The model under review builds one solid part; all positions refer to its coordinate system, in mm. A direction names the side the tool comes from. Give positions to 0.01 mm unless a question says otherwise; leave off trailing zeros. Order: outer loops, then holes, each group sorted by start corner. A loop starts at its lowest first (then second) coordinate and runs counter-clockwise, first axis right, second up.
```python
from build123d import *

# Parameters (mm, degrees)
BOSS_EXTRUDE11_DEPTH = 10
BOSS_EXTRUDE12_DEPTH = 2
BOSS_EXTRUDE15_START = -8
BOSS_EXTRUDE15_DEPTH = 2
BOSS_EXTRUDE19_START = -10
SKETCH1_20_W         = 1.25
SKETCH1_20_H         = 3.5
BOSS_EXTRUDE19_DEPTH = 10
BOSS_EXTRUDE20_START = -20
SKETCH1_21_W         = 197.5
SKETCH1_21_H         = 3.5
BOSS_EXTRUDE20_DEPTH = 2
CUT_EXTRUDE1_REACH   = 249.148
SKETCH2_R            = 2.5
SKETCH2_3_R          = 6
SKETCH2_3_R_2        = 2.5
CUT_EXTRUDE2_DEPTH   = 4.75
CUT_EXTRUDE3_REACH   = 249.625
SKETCH3_R            = 2.5
SKETCH3_3_R          = 6
SKETCH3_3_R_2        = 2.5
CUT_EXTRUDE4_DEPTH   = 4.75


with BuildPart() as part:
    # Sketch1 → Boss-Extrude11 (new body)
    with BuildSketch(Plane.XY):
        with BuildLine():
            Line((201.25, 4.75), (201.25, 27.25))
            Line((201.25, 27.25), (1.25, 27.25))
            Line((1.25, 27.25), (1.25, 30.75))
            Line((1.25, 30.75), (226.5, 30.75))
            ThreePointArc((226.5, 30.75), (243, 14.25), (226.5, -2.25))
            Line((226.5, -2.25), (210, -2.25))
            Line((210, -2.25), (210, -3.5))
            Line((210, -3.5), (244.25, -3.5))
            Line((244.25, -3.5), (244.25, 32))
            Line((244.25, 32), (0, 32))
            Line((0, 32), (0, 26))
            Line((0, 26), (200, 26))
            Line((200, 26), (200, 6))
            Line((200, 6), (0, 6))
            Line((0, 6), (0, 0))
            Line((0, 0), (208.75, 0))
            Line((208.75, 0), (208.75, 1.25))
            Line((208.75, 1.25), (1.25, 1.25))
            Line((1.25, 1.25), (1.25, 4.75))
            Line((1.25, 4.75), (201.25, 4.75))
        make_face()
    extrude(amount=-BOSS_EXTRUDE11_DEPTH)

    # Sketch1<12> → Boss-Extrude12 (add)
    with BuildSketch(Plane.XY):
        with BuildLine():
            Line((201.25, 4.75), (1.25, 4.75))
            Line((1.25, 4.75), (1.25, 1.25))
            Line((1.25, 1.25), (208.75, 1.25))
            Line((208.75, 1.25), (208.75, 0))
            Line((208.75, 0), (210, 0))
            Line((210, 0), (210, -2.25))
            Line((210, -2.25), (226.5, -2.25))
            ThreePointArc((226.5, -2.25), (210, 14.25), (226.5, 30.75))
            Line((226.5, 30.75), (1.25, 30.75))
            Line((1.25, 30.75), (1.25, 27.25))
            Line((1.25, 27.25), (201.25, 27.25))
            Line((201.25, 27.25), (201.25, 4.75))
        make_face()
    extrude(amount=-BOSS_EXTRUDE12_DEPTH)

    # Sketch1<14> → Boss-Extrude15 (add)
    with BuildSketch(Plane.XY.offset(BOSS_EXTRUDE15_START)):
        with BuildLine():
            Line((201.25, 4.75), (198.75, 4.75))
            Line((198.75, 4.75), (198.75, 1.25))
            Line((198.75, 1.25), (208.75, 1.25))
            Line((208.75, 1.25), (208.75, 0))
            Line((208.75, 0), (210, 0))
            Line((210, 0), (210, -2.25))
            Line((210, -2.25), (226.5, -2.25))
            ThreePointArc((226.5, -2.25), (243, 14.25), (226.5, 30.75))
            Line((226.5, 30.75), (198.75, 30.75))
            Line((198.75, 30.75), (198.75, 27.25))
            Line((198.75, 27.25), (201.25, 27.25))
            Line((201.25, 27.25), (201.25, 4.75))
        make_face()
    extrude(amount=-BOSS_EXTRUDE15_DEPTH)

    # Sketch1<20> → Boss-Extrude19 (add)
    with BuildSketch(Plane.XY.offset(BOSS_EXTRUDE19_START)):
        Polygon((0, 26), (200, 26), (200, 27.25), (198.75, 27.25), (1.25, 27.25), (1.25, 30.75), (198.75, 30.75), (200, 30.75), (200, 32), (0, 32), align=None)
        with Locations((199.375, 29)):
            Rectangle(SKETCH1_20_W, SKETCH1_20_H)
        with Locations((199.375, 3)):
            Rectangle(SKETCH1_20_W, SKETCH1_20_H)
        Polygon((200, 4.75), (200, 6), (0, 6), (0, 0), (200, 0), (200, 1.25), (198.75, 1.25), (1.25, 1.25), (1.25, 4.75), (198.75, 4.75), align=None)
    extrude(amount=-BOSS_EXTRUDE19_DEPTH)

    # Sketch1<21> → Boss-Extrude20 (add)
    with BuildSketch(Plane.XY.offset(BOSS_EXTRUDE20_START)):
        with Locations((100, 3)):
            Rectangle(SKETCH1_21_W, SKETCH1_21_H)
        with Locations((100, 29)):
            Rectangle(SKETCH1_21_W, SKETCH1_21_H)
    extrude(amount=BOSS_EXTRUDE20_DEPTH)

    # Cut-Extrude1: up to this face of the body (flat: up to its plane)
    cut_extrude1_end = Plane(part.part.faces().sort_by_distance((100, 6, -10))[0])
    # Sketch2 → Cut-Extrude1 (cut, up to the picked face)
    with BuildSketch(Plane.XZ, mode=Mode.PRIVATE) as cut_extrude1_sk1:
        with Locations((32.5, -10)):
            Circle(SKETCH2_R)
    cut_extrude1_tool1 = split(extrude(cut_extrude1_sk1.sketch, amount=-CUT_EXTRUDE1_REACH, mode=Mode.PRIVATE), bisect_by=cut_extrude1_end, keep=Keep.BOTH, mode=Mode.PRIVATE)
    # Sketch2 → Cut-Extrude1 (cut, up to the picked face)
    with BuildSketch(Plane.XZ, mode=Mode.PRIVATE) as cut_extrude1_sk2:
        with Locations((155, -10)):
            Circle(SKETCH2_R)
    cut_extrude1_tool2 = split(extrude(cut_extrude1_sk2.sketch, amount=-CUT_EXTRUDE1_REACH, mode=Mode.PRIVATE), bisect_by=cut_extrude1_end, keep=Keep.BOTH, mode=Mode.PRIVATE)
    add(cut_extrude1_tool1.solids().sort_by(Axis((32.5, 0, -10), (0, 1, 0)))[0], mode=Mode.SUBTRACT)
    add(cut_extrude1_tool2.solids().sort_by(Axis((155, 0, -10), (0, 1, 0)))[0], mode=Mode.SUBTRACT)

    # Sketch2<3> → Cut-Extrude2 (cut)
    # profile 1 of 2: a face of its own
    with BuildSketch(Plane.XZ):
        with Locations(Location((155, -10, 0), (0, 0, 270))):
            Circle(SKETCH2_3_R)
        with Locations((155, -10)):
            Circle(SKETCH2_3_R_2, mode=Mode.SUBTRACT)
    # profile 2 of 2: a face of its own
    with BuildSketch(Plane.XZ):
        with Locations(Location((32.5, -10, 0), (0, 0, 270))):
            Circle(SKETCH2_3_R)
        with Locations((32.5, -10)):
            Circle(SKETCH2_3_R_2, mode=Mode.SUBTRACT)
    extrude(amount=-CUT_EXTRUDE2_DEPTH, mode=Mode.SUBTRACT)

    # Cut-Extrude3: up to this face of the body (flat: up to its plane)
    cut_extrude3_end = Plane(part.part.faces().sort_by_distance((100, 26, -10))[0])
    # Sketch3 → Cut-Extrude3 (cut, up to the picked face)
    with BuildSketch(Plane(origin=(0, 32, 0), x_dir=(1, 0, 0), z_dir=(0, 1, 0)), mode=Mode.PRIVATE) as cut_extrude3_sk1:
        with Locations(Location((157.5, 10, 0), (0, 0, 180))):
            Circle(SKETCH3_R)
    cut_extrude3_tool1 = split(extrude(cut_extrude3_sk1.sketch, amount=-CUT_EXTRUDE3_REACH, mode=Mode.PRIVATE), bisect_by=cut_extrude3_end, keep=Keep.BOTH, mode=Mode.PRIVATE)
    # Sketch3 → Cut-Extrude3 (cut, up to the picked face)
    with BuildSketch(Plane(origin=(0, 32, 0), x_dir=(1, 0, 0), z_dir=(0, 1, 0)), mode=Mode.PRIVATE) as cut_extrude3_sk2:
        with Locations(Location((55, 10, 0), (0, 0, 180))):
            Circle(SKETCH3_R)
    cut_extrude3_tool2 = split(extrude(cut_extrude3_sk2.sketch, amount=-CUT_EXTRUDE3_REACH, mode=Mode.PRIVATE), bisect_by=cut_extrude3_end, keep=Keep.BOTH, mode=Mode.PRIVATE)
    add(cut_extrude3_tool1.solids().sort_by(Axis((157.5, 32, -10), (0, -1, 0)))[0], mode=Mode.SUBTRACT)
    add(cut_extrude3_tool2.solids().sort_by(Axis((55, 32, -10), (0, -1, 0)))[0], mode=Mode.SUBTRACT)

    # Sketch3<3> → Cut-Extrude4 (cut)
    # profile 1 of 2: a face of its own
    with BuildSketch(Plane(origin=(0, 32, 0), x_dir=(1, 0, 0), z_dir=(0, 1, 0))):
        with Locations(Location((157.5, 10, 0), (0, 0, 180))):
            Circle(SKETCH3_3_R)
        with Locations(Location((157.5, 10, 0), (0, 0, 180))):
            Circle(SKETCH3_3_R_2, mode=Mode.SUBTRACT)
    # profile 2 of 2: a face of its own
    with BuildSketch(Plane(origin=(0, 32, 0), x_dir=(1, 0, 0), z_dir=(0, 1, 0))):
        with Locations(Location((55, 10, 0), (0, 0, 180))):
            Circle(SKETCH3_3_R)
        with Locations(Location((55, 10, 0), (0, 0, 180))):
            Circle(SKETCH3_3_R_2, mode=Mode.SUBTRACT)
    extrude(amount=-CUT_EXTRUDE4_DEPTH, mode=Mode.SUBTRACT)


solid = part.part
```
1. Take a section at A-A (x = 55). Write out the cut boundary in (y, z).
2. Take a section at C-C (y = 14.25). Write out the cut boundary in (x, z), and give its area (3 significant figures).
3. Take a section at B-B (x = 175). Write out the cut boundary in (y, z), and give its area (3 significant figures).
4. Draft analysis for pull direction Z (two halves, no side actions). For faces 1 (the flat face through (104, 0, -10)), 2 (the flat face through (222, 14, -10)), 3 (the cylindrical face through (155.19, 26.63, -10.96)), 4 (the flat face through (221, 14, -8)), state which applies: pulls with the +Z half, pulls with the -Z half, needs draft (parallel to the pull), parting line crosses it, or undercut.
5. For faces 5 (the cylindrical face through (31.96, 5.37, -12.44)), 6 (the cylindrical face through (61, 31, -10)), 7 (the flat face through (103, 27.25, -10)), list the 3-axis set-ups (+Z, -Z, +X, -X, +Y, -Y) from which the entire face can be reached by the end or side of a thin tool; tool diameter is ignored.
6. To check wall thickness, follow line 1 (Y direction, x = 84, z = -15.75); line 2 (Y direction, x = 149.5, z = -8.5); line 3 (Y direction, x = 29.5, z = -18.75). State the ranges of each line that lie inside material, in increasing order.
7. Insertion check: pin 1 (8 mm diameter, centred on x = 43.5, z = -10, fed in from -Y); pin 2 (1.5 mm diameter, centred on y = 5.5, z = -10.5, fed in from -X); pin 3 (1.8 mm diameter, centred on y = 28.5, z = -12, fed in from +X); pin 4 (11 mm diameter, centred on x = 155, z = -10, fed in from -Y). Each pin has a flat end and moves straight along its axis. Give the tip position at first contact, or say it passes through.
Answer:
1. outline: (0, -20) - (6, -20) - (6, 0) - (0, 0) - close; (26, -20) - (32, -20) - (32, -16) - (30.75, -16) - (30.75, -18) - (27.25, -18) - (27.25, -12.5) - (26, -12.5) - close; (26, -7.5) - (27.25, -7.5) - (27.25, -2) - (30.75, -2) - (30.75, -4) - (32, -4) - (32, 0) - (26, 0) - close; hole (1.25, -18) - (4.75, -18) - (4.75, -2) - (1.25, -2) - close
2. outline: (200, -10) - (244.25, -10) - (244.25, 0) - (243, 0) - (243, -8) - (201.25, -8) - (201.25, -2) - (210, -2) - (210, 0) - (200, 0) - close
2. area: 126 mm2
3. outline: (0, -20) - (6, -20) - (6, 0) - (0, 0) - close; (26, -20) - (32, -20) - (32, 0) - (26, 0) - close; hole (1.25, -18) - (4.75, -18) - (4.75, -2) - (1.25, -2) - close; hole (27.25, -18) - (30.75, -18) - (30.75, -2) - (27.25, -2) - close
3. area: 128 mm2
4. face 1: needs draft
4. face 2: pulls with the -Z half
4. face 3: undercut
4. face 4: undercut
5. face 5: -Y
5. face 6: +Y
5. face 7: none
6. line 1: y = 0 to 1.25, 4.75 to 6, 26 to 27.25, 30.75 to 32
6. line 2: y = 4.75 to 6, 26 to 27.25, 30.75 to 32
6. line 3: y = 0 to 6, 26 to 32
7. pin 1: stops at y = 0
7. pin 2: stops at x = 0
7. pin 3: stops at x = 200
7. pin 4: stops at y = 4.75
